Build history of the part. All positions in model axes, mm. Give positions to 0.01 mm unless a question says otherwise; leave off trailing zeros. Write each loop counter-clockwise with the first axis right and the second up, starting at its lowest first coordinate (ties: lowest second). Pieces come first, ordered by that corner, then holes. Notation, with made-up numbers: (77, -18.5) -> (100, -18.5) arc R18 ccw to (100, -0.5) -> close; hole circle Ø6 at (-25.5, -8.75). An arc over 180 degrees is marked (long way). Put each result on its own line as item: value.
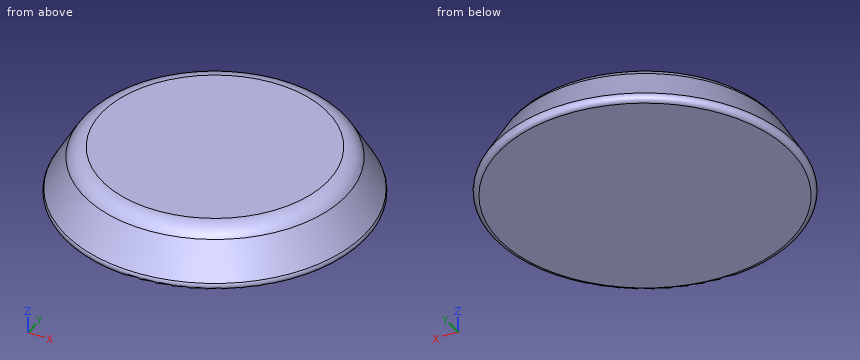
from build123d import *

# Parameters (mm, degrees)
F0_R     = 19.05
F1_DEPTH = 6.35
F1_TAPER = 30
F2_R     = 2.54
F3_R     = 0.635


with BuildPart() as f1:
    # F0 (on Top) → F1 (new body)
    with BuildSketch(Plane.XY):
        Circle(F0_R)
    extrude(amount=F1_DEPTH, taper=F1_TAPER)

    # F2
    f2_edges = [f1.edges().sort_by_distance(p)[0] for p in [
        (-15.383826, 0, 6.35),
    ]]
    fillet(f2_edges, radius=F2_R)

    # F3
    f3_edges = [f1.edges().sort_by_distance(p)[0] for p in [
        (-19.05, 0, 0),
    ]]
    fillet(f3_edges, radius=F3_R)


solid = f1.part
1) Wall check: L1, parallel to X at y = -5.5, z = 3.5; L2, parallel to X at y = -11, z = 3.5; L3, parallel to Z at x = 12, y = 11.5. Give the ranges that are in metal, low to high.
Filled sheet:
L1: -16.12 to 16.12
L2: -13 to 13
L3: 0 to 4.21
2) Slice it at D-D (z = 0.5). Write the cut outline in (x, y).
Filled sheet:
outline: circle Ø37.14 at (0, 0)
3) Slice it at C-C (z = 2.75). Write the cut outline in (x, y).
Filled sheet:
outline: circle Ø34.92 at (0, 0)
4) Pin check, flat tips, straight feed: pin 1 (5 mm diameter, centred on x = -0.5, y = -4, fed in from -Z); pin 2 (2 mm diameter, centred on x = 0, z = 5.5, fed in from +Y); pin 3 (1.5 mm diameter, centred on x = 2.5, z = 5.5, fed in from -Y). Stop position of each tip, or through.
Filled sheet:
pin 1: z = 0
pin 2: y = 16.45
pin 3: y = -16.13
